Read the model definition and answer for the solid it produces. Units are mm, in the model's axes. Face numbers are marked on the shaded views. A direction names the side the tool comes from. Coordinates: 2 decimals unless noted, no trailing zeros. Write each loop counter-clockwise with the first axis right and the second up, starting at its lowest first coordinate (ties: lowest second). Pieces come first, ordered by that corner, then holes. Notation, with made-up numbers: (85.25, -6.5) - (118.25, -6.5) arc R33 ccw to (118.25, 31.5) - close; hole circle Ø10 at (72, -10). An arc over 180 degrees is marked (long way). Use a Markdown table: item, result.
from build123d import *

# Parameters (mm, degrees)
F1_DEPTH = 5.55625
F2_R     = 1.2192
F3_DEPTH = 25.4
F4_R     = 1.1303
F5_DEPTH = 25.4
F6_R     = 2.778115
F7_R     = 2.778115
F8_R     = 1.1303
F9_DEPTH = 25.4


# Not quite as in the source:
# - a fillet or chamfer is up to 0.001 mm smaller than in the source, because OpenCascade refuses the exact size
# - ends of sketch curves that miss each other by under 0.0002 mm in the source are joined


with BuildPart() as f1:
    # F0 (on Top) → F1 (new body)
    with BuildSketch(Plane.XY):
        with BuildLine():
            Line((29.0973595662, 23.0125838354), (-28.0526404338, 23.0125838354))
            Line((-28.0526404338, 23.0125838354), (-28.0526404338, 20.6313338354))
            Line((-28.0526404338, 20.6313338354), (29.0973595662, 20.6313338354))
            ThreePointArc((29.0973595662, 20.6313338354), (29.6586255738, 20.398849843), (29.8911095662, 19.8375838354))
            Line((29.8911095662, 19.8375838354), (29.8911095662, 19.4407088354))
            ThreePointArc((29.8911095662, 19.4407088354), (30.1235935587, 18.8794428278), (30.6848595662, 18.6469588354))
            Line((30.6848595662, 18.6469588354), (44.9723595662, 18.6469588354))
            Line((44.9723595662, 18.6469588354), (44.9723595662, 20.2344588354))
            Line((44.9723595662, 20.2344588354), (32.2723595662, 20.2344588354))
            Line((32.2723595662, 20.2344588354), (32.2723595662, 23.4094588354))
            Line((32.2723595662, 23.4094588354), (44.9723595662, 23.4094588354))
            Line((44.9723595662, 23.4094588354), (44.9723595662, 24.9969588354))
            Line((44.9723595662, 24.9969588354), (30.6848595662, 24.9969588354))
            ThreePointArc((30.6848595662, 24.9969588354), (30.1235935587, 24.764474843), (29.8911095662, 24.2032088354))
            Line((29.8911095662, 24.2032088354), (29.8911095662, 23.8063338354))
            ThreePointArc((29.8911095662, 23.8063338354), (29.6586255738, 23.2450678278), (29.0973595662, 23.0125838354))
        make_face()
    extrude(amount=F1_DEPTH)

    # F2 (on face) → F3 (cut)
    with BuildSketch(Plane.XZ.offset(-20.6313338354)):
        with Locations((-25.2745154338, 2.778125)):
            Circle(F2_R)
    extrude(amount=-F3_DEPTH, mode=Mode.SUBTRACT)

    # F4 (on face) → F5 (cut)
    with BuildSketch(Plane.XZ.offset(-18.6469588354)):
        with Locations((42.1942345662, 2.778125)):
            Circle(F4_R)
    extrude(amount=-F5_DEPTH, mode=Mode.SUBTRACT)

    # F6 (radius 2.778125 in the source; OpenCascade refuses exactly that, so slightly less here)
    f6_edges = [f1.edges().sort_by_distance(p)[0] for p in [
        (44.97236, 19.440709, 5.55625),
        (44.97236, 19.440709, 0),
        (44.97236, 24.203209, 0),
        (44.97236, 24.203209, 5.55625),
    ]]
    fillet(f6_edges, radius=F6_R)

    # F7 (radius 2.778125 in the source; OpenCascade refuses exactly that, so slightly less here)
    f7_edges = [f1.edges().sort_by_distance(p)[0] for p in [
        (-28.05264, 21.821959, 5.55625),
        (-28.05264, 21.821959, 0),
    ]]
    fillet(f7_edges, radius=F7_R)

    # F8 (on face) → F9 (cut)
    with BuildSketch(Plane.XZ.offset(-20.6313338354)):
        with Locations((8.0629845662, 2.778125)):
            Circle(F8_R)
        with BuildLine():
            Line((8.0629845662, 5.55625), (-25.2745254338, 5.55625))
            ThreePointArc((-25.2745254338, 5.55625), (-24.3987826977, 5.4146133255), (-23.612344628, 5.0041453791))
            ThreePointArc((-23.612344628, 5.0041453791), (-22.6534079634, 4.515722008), (-21.5864000573, 4.375682569))
            Line((-21.5864000573, 4.375682569), (8.0629845662, 5.55625))
        make_face()
        with BuildLine():
            ThreePointArc((-23.6851494527, 0.4995521366), (-24.4415033451, 0.1278289079), (-25.2745154338, 0))
            Line((-25.2745154338, 0), (8.0629845662, 0))
            Line((8.0629845662, 0), (-21.7550382738, 1.0684326083))
            ThreePointArc((-21.7550382738, 1.0684326083), (-22.7663528525, 0.9409409702), (-23.6851494527, 0.4995521366))
        make_face()
    extrude(amount=-F9_DEPTH, mode=Mode.SUBTRACT)


solid = f1.part
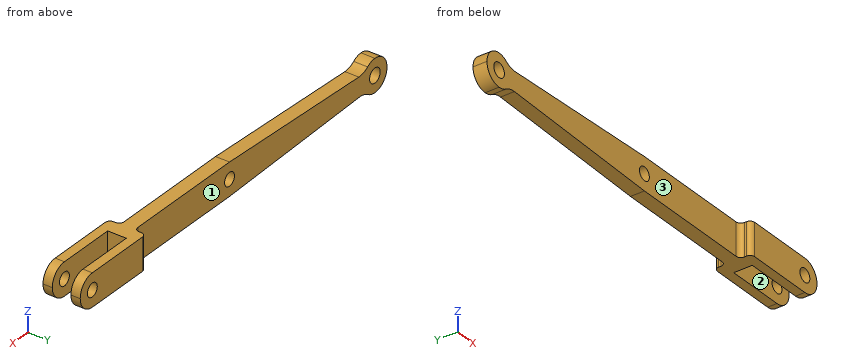
(1) A cutting plane is placed at A-A, the plane x = 23.5. Write down the section's boundary in (y, z).
Report:
| item | result |
|---|---|
| outline | (20.63, 0) - (23.01, 0) - (23.01, 5.56) - (20.63, 5.56) - close |
(2) For the marked faces 1, 2 and 3, determine the directions among +Z, -Z, +X, -X, +Y, -Y from which every point of the face is accessible in a straight line to the end or side of a thin tool.
Report:
| item | result |
|---|---|
| face 1 | +Z, -Z, -X, +Y |
| face 2 | +Z, -Z, +X |
| face 3 | +Z, -Z, -X, -Y |
(3) Each of these flat-tipped pins is pushed along its axis until it touches: P1, Ø1.5, axis at y = 22.5, z = 3, coming from the +X side; P2, Ø1, axis at x = 1, y = 21.5, coming from the -Z side; P3, Ø3, axis at x = -25.27, z = 2.78, coming from the +Y side; P4, Ø1.4, axis at x = 42.19, z = 2.78, coming from the +Y side. Where does it stop, or does it pass through?
Report:
| item | result |
|---|---|
| P1 | stops at x = 32.27 |
| P2 | stops at z = 0.24 |
| P3 | stops at y = 23.01 |
| P4 | passes through |
(4) A cutting plane is placed at B-B, the plane x = 3.5. Write down the section's boundary in (y, z), and give its area (3 significant figures).
Report:
| item | result |
|---|---|
| outline | (20.63, 0.16) - (23.01, 0.16) - (23.01, 5.37) - (20.63, 5.37) - close |
| area | 12.4 mm² |
(5) Straight lines are drawn through the part: L1, parallel to X at y = 21.75, z = 2.4; L2, parallel to X at y = 21, z = 2.55; L3, parallel to Y at x = 41, z = 1.65. For each, find the intervals that lie inside material, in ascending order.
Report:
| item | result |
|---|---|
| L1 | x = -28.03 to -26.43, -24.12 to 7, 9.13 to 32.27 |
| L2 | x = -28.04 to -26.47, -24.08 to 6.96, 9.17 to 32.27 |
| L3 | y = 18.65 to 20.23, 23.41 to 25 |
